Source: CAD feature listing. Evaluate the final solid. Frame: model axes, mm. Face numbers are marked on the shaded views. A direction names the side the tool comes from. Coordinates: 2 decimals unless noted, no trailing zeros. Order: outer loops, then holes, each group sorted by start corner. A loop starts at its lowest first (then second) coordinate and runs counter-clockwise, first axis right, second up.
```python
from build123d import *


with BuildPart() as part:
    # Sketch → Revolution (revolve)
    with BuildSketch(Plane.XZ):
        Polygon((-9, 0), (-11, 0), (-11, 6.5), (-5.2, 12.3), (-4, 14), (-4, 20.3), (-5, 20.3), (-4, 28.3), (-5, 28.3), (-4, 36.3), (-3.2, 36.3), (-3.2, 12.3), (-9, 6.5), align=None)
    revolve(axis=Axis((0, 0, 0), (0, 0, 1)))


solid = part.part
```
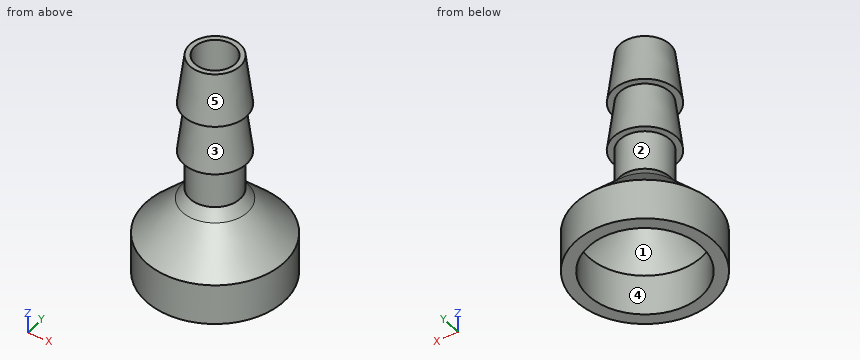
1. Section query A-A, the plane y = 0. Output: boundary loops of the cut face in (x, z), plus the area to 3 significant figures.
2. Draft query along X for the marked faces 1 and 2. Return one class per face: +X half, -X half, draft (parallel to the pull), parting line (faces both ways), or undercut.
3. Section query C-C, the plane z = 9. Output: boundary loops of the cut face in (x, y).
4. Material intervals for line 1 along X through (y, z) = (0, 3); line 2 along X through (y, z) = (2.25, 11.5), sorted ascending.
5. Contact query for flat-ended pins moving along their axis: P1, Ø1.5, axis at x = -1, y = 6, coming from the +Z side; P2, Ø2, axis at y = 0, z = 30.5, coming from the -X side; P3, Ø3, axis at x = -4.5, z = 9, coming from the +Y side; P4, Ø2, axis at x = -5.5, y = -8.5, coming from the -Z side. Output: stop coordinate, or through.
6. Section query D-D, the plane x = 4.5. Count the separate pieces of the cut face and the enclosed holes in it, plus the area to 3 significant figures.
7. Access query for the marked faces 3, 4 and 5. Directions: +Z, -Z, +X, -X, +Y, -Y. A direction counts if a zero-diameter tool reaches every point of the face in a straight line with its end or side. Return the directions, or none.
Answer key:
1. outline: (-11, 0) - (-9, 0) - (-9, 6.5) - (-3.2, 12.3) - (-3.2, 36.3) - (-4, 36.3) - (-5, 28.3) - (-4, 28.3) - (-5, 20.3) - (-4, 20.3) - (-4, 14) - (-5.2, 12.3) - (-11, 6.5) - close; (3.2, 12.3) - (9, 6.5) - (9, 0) - (11, 0) - (11, 6.5) - (5.2, 12.3) - (4, 14) - (4, 20.3) - (5, 20.3) - (4, 28.3) - (5, 28.3) - (4, 36.3) - (3.2, 36.3) - close
1. area: 106 mm2
2. face 1: undercut
2. face 2: parting line
3. outline: circle Ø17 at (0, 0); hole circle Ø13 at (0, 0)
4. line 1: x = -11 to -9, 9 to 11
4. line 2: x = -5.56 to -3.31, 3.31 to 5.56
5. P1: stops at z = 12.17
5. P2: stops at x = -4.85
5. P3: stops at y = 9.07
5. P4: stops at z = 0
6. separate pieces: 3
6. enclosed holes: 0
6. area: 88.9 mm2
7. face 3: none
7. face 4: -Z
7. face 5: +Z
